Work out the finished part from the listing and answer in its coordinate system (mm). Coordinates: 2 decimals unless noted, no trailing zeros. Loops run counter-clockwise (first coordinate to the right, second up) from the corner with the lowest first, then second, coordinate; pieces in that order, holes last.
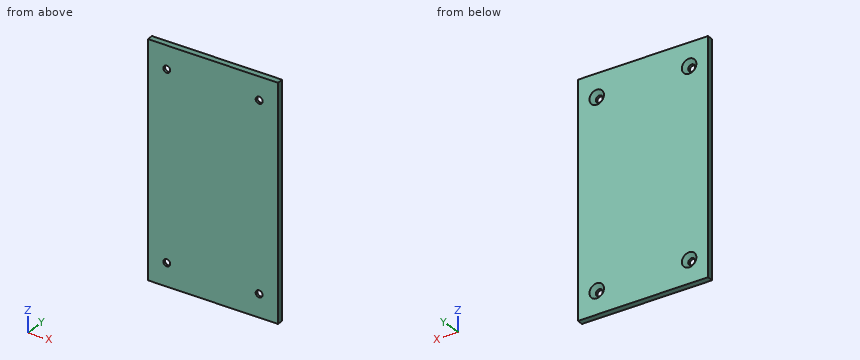
```python
from build123d import *

# Parameters (mm, degrees)
SKETCH1_W                                      = 84.5
SKETCH1_H                                      = 149.5
BASE_FLANGE1_DEPTH                             = 4
CSK_FOR_M4_FLAT_HEAD_MACHINE_SCREW1_AT_2_COUNT = 2
CSK_FOR_M4_FLAT_HEAD_MACHINE_SCREW1_AT_2_PITCH = 60
CSK_FOR_M4_FLAT_HEAD_MACHINE_SCREW1_AT_3_COUNT = 2
CSK_FOR_M4_FLAT_HEAD_MACHINE_SCREW1_AT_3_PITCH = 134.16407865
CSK_FOR_M4_FLAT_HEAD_MACHINE_SCREW1_AT_4_COUNT = 2
CSK_FOR_M4_FLAT_HEAD_MACHINE_SCREW1_AT_4_PITCH = 120


# Sheet-metal steps are written as plain solids
with BuildPart() as part:
    # Sketch1 → Base-Flange1 (new body)
    with BuildSketch(Plane(origin=(0, 0, 0), x_dir=(1, 0, 0), z_dir=(0, 1, 0))):
        Rectangle(SKETCH1_W, SKETCH1_H)
    extrude(amount=-BASE_FLANGE1_DEPTH)

    # Sketch5 → CSK for M4 Flat Head Machine Screw1 (revolve, cut)
    with BuildSketch(Plane(origin=(30, 0, -60), x_dir=(0, 0, 1), z_dir=(1, 0, 0))):
        Polygon((0, 0), (0, 4), (2.25, 4), (2.25, 2.45), (4.7, 0), align=None)
    csk_for_m4_flat_head_machine_screw1 = revolve(axis=Axis((30, 6.35, -60), (0, -1, 0)), mode=Mode.SUBTRACT)

    # CSK for M4 Flat Head Machine Screw1 at 2: CSK for M4 Flat Head Machine Screw1 ×2
    with Locations(*[(-i * CSK_FOR_M4_FLAT_HEAD_MACHINE_SCREW1_AT_2_PITCH, 0, 0) for i in range(1, CSK_FOR_M4_FLAT_HEAD_MACHINE_SCREW1_AT_2_COUNT)]):
        add(csk_for_m4_flat_head_machine_screw1, mode=Mode.SUBTRACT)

    # CSK for M4 Flat Head Machine Screw1 at 3: CSK for M4 Flat Head Machine Screw1 ×2
    with Locations(*[Vector(-0.44721359549995787, 0, 0.894427190999916) * (i * CSK_FOR_M4_FLAT_HEAD_MACHINE_SCREW1_AT_3_PITCH) for i in range(1, CSK_FOR_M4_FLAT_HEAD_MACHINE_SCREW1_AT_3_COUNT)]):
        add(csk_for_m4_flat_head_machine_screw1, mode=Mode.SUBTRACT)

    # CSK for M4 Flat Head Machine Screw1 at 4: CSK for M4 Flat Head Machine Screw1 ×2
    with Locations(*[(0, 0, i * CSK_FOR_M4_FLAT_HEAD_MACHINE_SCREW1_AT_4_PITCH) for i in range(1, CSK_FOR_M4_FLAT_HEAD_MACHINE_SCREW1_AT_4_COUNT)]):
        add(csk_for_m4_flat_head_machine_screw1, mode=Mode.SUBTRACT)


solid = part.part
```
1. Straight lines are drawn through the part: probe 1 along X at (y, z) = (-3.25, 60); probe 2 along Z at (x, y) = (30, -2.75); probe 3 along Z at (x, y) = (30.5, -1). For each, find the intervals that lie inside material, in ascending order.
2. A cutting plane is placed at B-B, the plane x = 30. Give the vertices of the cut face in (y, z).
3. A cutting plane is placed at A-A, the plane z = -60. Give the vertices of the cut face in (x, y), then the cut area to 3 significant figures.
4. This flat-tipped pin is pushed along its axis until it touches: P1, Ø3.5, axis at x = 30, z = -60, coming from the -Y side. Where does it stop, or does it pass through?
Answers below:
1. probe 1: x = -42.25 to -32.25, -27.75 to 27.75, 32.25 to 42.25
1. probe 2: z = -74.75 to -62.25, -57.75 to 57.75, 62.25 to 74.75
1. probe 3: z = -74.75 to -63.67, -56.33 to 56.33, 63.67 to 74.75
2. outline: (-4, -74.75) - (0, -74.75) - (0, -64.7) - (-2.45, -62.25) - (-4, -62.25) - close; (-4, -57.75) - (-2.45, -57.75) - (0, -55.3) - (0, 55.3) - (-2.45, 57.75) - (-4, 57.75) - close; (-4, 62.25) - (-2.45, 62.25) - (0, 64.7) - (0, 74.75) - (-4, 74.75) - close
3. outline: (-42.25, -4) - (-32.25, -4) - (-32.25, -2.45) - (-34.7, 0) - (-42.25, 0) - close; (-27.75, -4) - (27.75, -4) - (27.75, -2.45) - (25.3, 0) - (-25.3, 0) - (-27.75, -2.45) - close; (32.25, -4) - (42.25, -4) - (42.25, 0) - (34.7, 0) - (32.25, -2.45) - close
3. area: 290 mm2
4. P1: passes through
